Can you work these out from the model? Positions are in its coordinate system, mm. Face numbers are marked on the shaded views. A direction names the side the tool comes from. Give positions to 0.01 mm unless a question says otherwise; leave off trailing zeros. Write each loop counter-clockwise with the first axis right and the second up, starting at its lowest first coordinate (ties: lowest second). Pieces come first, ordered by that corner, then holes. Notation, with made-up numbers: M 24.25,23 L 76.25,23 A22 ccw 76.25,60 Z; hole C 7,44.5 d7. An arc over 180 degrees is marked long. Write each question's results on one line, items separated by ' | '.
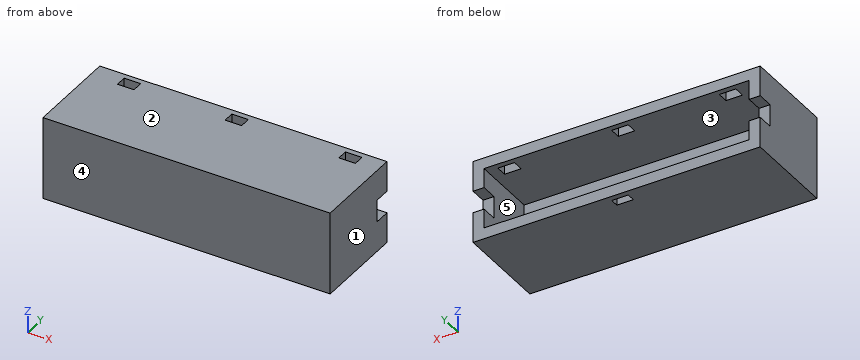
from build123d import *

# Parameters (mm, degrees)
SKETCH_1_W           = 520
SKETCH_1_H           = 150
EXTRUDE_1_DEPTH      = 140
SKETCH_2_W           = 480
SKETCH_2_H           = 110
CUT_EXTRUDE_1_DEPTH  = 120
SKETCH_11_W          = 40
SKETCH_11_H          = 30
CUT_EXTRUDE_3_DEPTH  = 544.714079273
SKETCH_13_W          = 520
SKETCH_13_H          = 150
EXTRUDE_6_DEPTH      = 30
SKETCH_18_W          = 30
SKETCH_18_H          = 15.352958973
CUT_EXTRUDE_8_DEPTH  = 30
SKETCH_21_W          = 30
SKETCH_21_H          = 19.875616275
CUT_EXTRUDE_9_DEPTH  = 30
SKETCH_22_W          = 30
SKETCH_22_H          = 19.88
CUT_EXTRUDE_10_DEPTH = 30
SKETCH_25_W          = 30
SKETCH_25_H          = 19.88
CUT_EXTRUDE_12_DEPTH = 30


with BuildPart() as part:
    # 草圖1 → 填料-伸長1 (new body)
    with BuildSketch(Plane(origin=(0, 0, 0), x_dir=(1, 0, 0), z_dir=(0, 1, 0))):
        Rectangle(SKETCH_1_W, SKETCH_1_H)
    extrude(amount=EXTRUDE_1_DEPTH)

    # 草圖2 → 除料-伸長1 (cut)
    with BuildSketch(Plane(origin=(0, 140, 0), x_dir=(1, 0, 0), z_dir=(0, 1, 0))):
        Rectangle(SKETCH_2_W, SKETCH_2_H)
    extrude(amount=-CUT_EXTRUDE_1_DEPTH, mode=Mode.SUBTRACT)

    # 草圖11 → 除料-伸長3 (cut, through all)
    with BuildSketch(Plane.ZY.offset(260)):
        with Locations((0, 125)):
            Rectangle(SKETCH_11_W, SKETCH_11_H)
    extrude(amount=-CUT_EXTRUDE_3_DEPTH, mode=Mode.SUBTRACT)

    # 草圖13 → 填料-伸長6 (add)
    with BuildSketch(Plane.XZ):
        Rectangle(SKETCH_13_W, SKETCH_13_H)
    extrude(amount=EXTRUDE_6_DEPTH)

    # 草圖18 → 除料-伸長8 (cut)
    with BuildSketch(Plane(origin=(0, 0, -75), x_dir=(-1, 0, 0), z_dir=(0, 0, -1))):
        with Locations((0, 122.323520514)):
            Rectangle(SKETCH_18_W, SKETCH_18_H)
    extrude(amount=-CUT_EXTRUDE_8_DEPTH, mode=Mode.SUBTRACT)

    # 草圖21 → 除料-伸長9 (cut)
    with BuildSketch(Plane.XY.offset(75)):
        with Locations((-195, 120.062191863)):
            Rectangle(SKETCH_21_W, SKETCH_21_H)
    extrude(amount=-CUT_EXTRUDE_9_DEPTH, mode=Mode.SUBTRACT)

    # 草圖22 → 除料-伸長10 (cut)
    with BuildSketch(Plane.XY.offset(75)):
        with Locations((0, 120.06)):
            Rectangle(SKETCH_22_W, SKETCH_22_H)
    extrude(amount=-CUT_EXTRUDE_10_DEPTH, mode=Mode.SUBTRACT)

    # 草圖25 → 除料-伸長12 (cut)
    with BuildSketch(Plane.XY.offset(75)):
        with Locations((205.891066665, 120.06)):
            Rectangle(SKETCH_25_W, SKETCH_25_H)
    extrude(amount=-CUT_EXTRUDE_12_DEPTH, mode=Mode.SUBTRACT)


solid = part.part
Item 1: If I drill on line 1 (X direction, y = 129.5, z = 55.5); line 2 (X direction, y = 100, z = 45); line 3 (Z direction, x = 15.5, y = 131.5), over which ranges is the centre line in solid material (lowest first)? Write a range as from..to.
Geometry says:
line 1: x = -260..-210, -180..-15, 15..190.89, 220.89..260 | line 2: x = -260..-240, 240..260 | line 3: z = -75..-55, 55..75
Item 2: For the marked faces 4 and 5, which set-ups out of +Z, -Z, +X, -X, +Y, -Y let a thin tool reach every point of the face, with its end or its side?
Geometry says:
face 4: +Z, -Z, +X, -X, -Y | face 5: +Y
Item 3: Thinking about a two-plate mould opening in Z: for the marked faces 1, 2 and 3, which applies, +Z half, -Z half, draft (parallel to the pull), parting line (faces both ways), or undercut?
Geometry says:
face 1: draft | face 2: +Z half | face 3: undercut
Item 4: I want a section at A-A, the plane y = 35. Please give me the cut outline in (x, z).
Geometry says:
outline: M -260,-75 L 260,-75 L 260,75 L -260,75 Z; hole M -240,-55 L 240,-55 L 240,55 L -240,55 Z
Item 5: I want a section at B-B, the plane x = -194.5. Please give me the cut outline in (y, z).
Geometry says:
outline: M -30,-75 L 140,-75 L 140,-55 L 20,-55 L 20,55 L 110.12,55 L 110.12,75 L -30,75 Z; M 130,55 L 140,55 L 140,75 L 130,75 Z
Item 6: I want a section at D-D, the plane x = 136. Please give me the cut outline in (y, z), and give its area (3 significant figures).
Geometry says:
outline: M -30,-75 L 140,-75 L 140,-55 L 20,-55 L 20,55 L 140,55 L 140,75 L -30,75 Z | area: 12,300 mm2
Item 7: I'm going to push flat-ended pins straight in: pin 1 (10 mm diameter, centred on x = 250.5, z = -5, fed in from +Y); pin 2 (8 mm diameter, centred on x = 4.5, z = -24.5, fed in from +Y). Where does each tip first touch, or does it pass through?
Geometry says:
pin 1: stops at y = 110 | pin 2: stops at y = 20
Item 8: I want a section at C-C, the plane y = 121. Give the number of separate pieces and of enclosed holes in the cut face, and give its area (3 significant figures).
Geometry says:
separate pieces: 6 | enclosed holes: 0 | area: 21,200 mm2
